Autodesk Inventor part; units mm, degrees
ref_plane "YZ Plane" through (0, 0, 0) normal (1, 0, 0) x (0, 1, 0)
ref_plane "XZ Plane" through (0, 0, 0) normal (0, 1, 0) x (-1, 0, 0)
ref_plane "XY Plane" through (0, 0, 0) normal (0, 0, 1) x (1, 0, 0)
sketch "スケッチ2" plane through (0, 0, 0) normal (0, 0, 1) x (1, 0, 0)
  line L0 (-31.5, 15) -> (31.5, 15)
  line L1 (31.5, 15) -> (31.5, -15)
  line L2 (31.5, -15) -> (-31.5, -15)
  line L3 (-31.5, -15) -> (-31.5, 15)
  line L4 (0, 24.6) -> (0, -21.6) construction
  line L5 (-44.1, 0) -> (44.1, 0) construction
  line L6 (-31.5, 15) -> (31.5, 15)
  line L7 (31.5, 15) -> (31.5, 18)
  line L8 (31.5, 18) -> (-31.5, 18)
  line L9 (-31.5, 18) -> (-31.5, 15)
  point P0 (0, 0)
  point P1 (31.5, 15)
  dimension "d1" = 63
  dimension "d2" = 30
  dimension "d3" = 15
  dimension "d4" = 31.5
  dimension "d26" = 3
extrude "押し出し1" add sketch "スケッチ2" along normal blind 3 contours L0 L1 L2 L3
sketch "スケッチ3" plane through (0, 0, 3) normal (0, 0, 1) x (1, 0, 0)
  line L0 (-31.5, -15) -> (31.5, -15) construction
  line L1 (-44.1, 0) -> (44.1, 0) construction
  line L2 (31.5, -15) -> (31.5, 15)
  line L3 (31.5, 15) -> (-31.5, 15)
  line L4 (-31.5, 15) -> (-31.5, -15)
  point P0 (0, 0)
  point P1 (-16.5, 0)
  point P2 (16.5, 0)
hole "穴1" at (-16.5, 0, 3) at (16.5, 0, 3) direction (0, 0, -1) diameter 6.6 end through all
fillet "フィレット1" radius 2 4 edges at (31.5, -15, 1.5) (-31.5, -15, 1.5) (-31.5, 15, 1.5) (31.5, 15, 1.5)
sketch "スケッチ4" plane through (0, 0, 3) normal (0, 0, 1) x (1, 0, 0)
  line L0 (-29.5, -15) -> (29.5, -15)
  arc A0 (-31.5, -13) -> (-29.5, -15) centre (-29.5, -13) ccw
  line L1 (-29.5, -15) -> (29.5, -15)
  arc A1 (29.5, -15) -> (31.5, -13) centre (29.5, -13) ccw
  circle A2 centre (-16.5, 0) radius 3.3
  circle A3 centre (16.5, 0) radius 3.3
  line L2 (1.5, -11) -> (-1.5, -11)
  line L3 (-1.5, -11) -> (-1.5, 11)
  line L4 (-1.5, 11) -> (1.5, 11)
  line L5 (1.5, 11) -> (1.5, -11)
  line L6 (1.5, -11) -> (-1.5, 11) construction
  line L7 (-1.5, -11) -> (1.5, 11) construction
  line L8 (31.5, -13) -> (31.5, 13)
  line L9 (29.5, 15) -> (-29.5, 15)
  line L10 (-31.5, 13) -> (-31.5, -13)
  arc A4 (31.5, 13) -> (29.5, 15) centre (29.5, 13) ccw
  arc A5 (-29.5, 15) -> (-31.5, 13) centre (-29.5, 13) ccw
  point P0 (0, 0)
  dimension "d22" = 3
  dimension "d24" = 4
extrude "押し出し2" add sketch "スケッチ4" along normal blind 3 contours L2 L3 L4 L5
fillet "フィレット2" radius 1 2 edges at (-1.5, 0, 6) (1.5, 0, 6)
fillet "フィレット2" radius 0.5 4 edges at (0, 11, 3) (0, -11, 3) (0, 11, 6) (0, -11, 6)
equation "\"d3\" = 0.5 * d2"
equation "\"d4\" = 0.5 * d1"
equation "\"d24\" = d23"
properties part number "rocker_frame_mount_00"
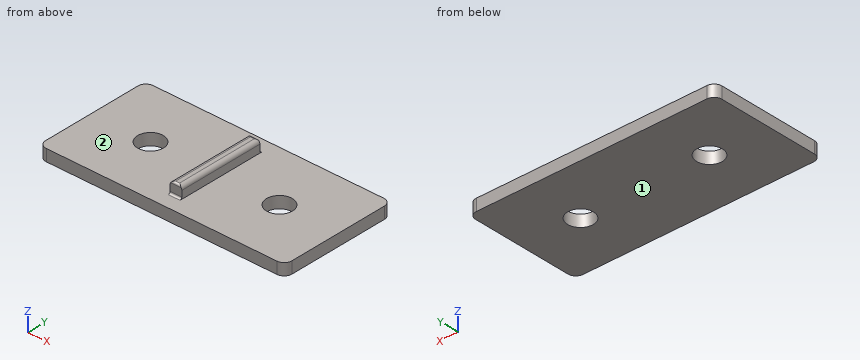
Here's how the part is built. I have some questions about the finished solid (model axes, mm). Face numbers are marked on the shaded views. Give positions to 0.01 mm unless a question says otherwise; leave off trailing zeros. Write each loop counter-clockwise with the first axis right and the second up, starting at its lowest first coordinate (ties: lowest second). Pieces come first, ordered by that corner, then holes. Notation, with made-up numbers: (52, -28) -> (90, -28) arc R22 ccw to (90, 5) -> close; hole circle Ø1 at (-1, 26.5). An arc over 180 degrees is marked (long way). Use one line per item in the form item = value. Start each with the question number.
1. Imagine slicing it at C-C on y = 0. List the corners of the cut face in (x, z) for me.
2. Imagine slicing it at D-D on y = 9.25. List the corners of the cut face in (x, z) for me.
3. Imagine slicing it at A-A on z = 2. List the corners of the cut face in (x, y) for me.
4. Imagine slicing it at B-B on x = -16.5. List the corners of the cut face in (y, z) for me.
5. If I drill on L1, parallel to X at y = 0, z = 1; L2, parallel to Y at x = -16.5, z = 1; L3, parallel to Z at x = 9.5, y = -0.75, over which ranges is the centre line in solid material (lowest first)?
6. Will these pins go through, and if not, where does the flat tip stop? pin 1 Ø1.5 at (x, y) = (-22.5, 8.5) entering from -Z; pin 2 Ø1.6 at (y, z) = (-1, 4.5) entering from +X; pin 3 Ø1 at (x, z) = (0.5, 5) entering from +Y; pin 4 Ø8.5 at (x, y) = (16.5, 0) entering from +Z.
7. Thinking about a two-plate mould opening in Z: for the marked faces 1 and 2, which applies, +Z half, -Z half, draft (parallel to the pull), parting line (faces both ways), or undercut?
Entries:
q1.outline = (-31.5, 0) -> (-19.8, 0) -> (-19.8, 3) -> (-31.5, 3) -> close; (-13.2, 0) -> (13.2, 0) -> (13.2, 3) -> (1.5, 3) -> (1.5, 5) arc R1 ccw to (0.5, 6) -> (-0.5, 6) arc R1 ccw to (-1.5, 5) -> (-1.5, 3) -> (-13.2, 3) -> close; (19.8, 0) -> (31.5, 0) -> (31.5, 3) -> (19.8, 3) -> close
q2.outline = (-31.5, 0) -> (31.5, 0) -> (31.5, 3) -> (1.5, 3) -> (1.5, 5) arc R1 ccw to (0.5, 6) -> (-0.5, 6) arc R1 ccw to (-1.5, 5) -> (-1.5, 3) -> (-31.5, 3) -> close
q3.outline = (-31.5, -13) arc R2 ccw to (-29.5, -15) -> (29.5, -15) arc R2 ccw to (31.5, -13) -> (31.5, 13) arc R2 ccw to (29.5, 15) -> (-29.5, 15) arc R2 ccw to (-31.5, 13) -> close; hole circle Ø6.6 at (-16.5, 0); hole circle Ø6.6 at (16.5, 0)
q4.outline = (-15, 0) -> (-3.3, 0) -> (-3.3, 3) -> (-15, 3) -> close; (3.3, 0) -> (15, 0) -> (15, 3) -> (3.3, 3) -> close
q5.L1 = -31.5 to -19.8, -13.2 to 13.2, 19.8 to 31.5
q5.L2 = -15 to -3.3, 3.3 to 15
q5.L3 = 0 to 3
q6.pin_1 = 0
q6.pin_2 = 1.5
q6.pin_3 = 11
q6.pin_4 = 3
q7.face_1 = -Z half
q7.face_2 = +Z half
